CAD build for the part. Positions are in the model's coordinates, mm. A direction names the side the tool comes from. Round coordinates to 2 decimals unless told otherwise and drop trailing zeros. Loops run counter-clockwise (first coordinate to the right, second up) from the corner with the lowest first, then second, coordinate; pieces in that order, holes last.
```python
from build123d import *

# Parameters (mm, degrees)
SKETCH1_W                        = 37
SKETCH1_H                        = 38
BOSS_EXTRUDE1_DEPTH              = 10
SKETCH2_W                        = 34
SKETCH2_H                        = 8
CUT_EXTRUDE1_DEPTH               = 38
CUT_EXTRUDE2_DEPTH               = 3
F_2_05_2_05_DIAMETER_HOLE1_D     = 2.05
F_2_05_2_05_DIAMETER_HOLE1_DEPTH = 10
F_10_0_10_DIAMETER_HOLE1_D       = 10
F_10_0_10_DIAMETER_HOLE1_DEPTH   = 10
F_2_7_2_7_DIAMETER_HOLE1_D       = 2.7
F_2_7_2_7_DIAMETER_HOLE1_DEPTH   = 2
F_2_7_2_7_DIAMETER_HOLE2_D       = 2.7
F_2_7_2_7_DIAMETER_HOLE2_DEPTH   = 2
F_2_7_2_7_DIAMETER_HOLE3_D       = 2.7
F_2_7_2_7_DIAMETER_HOLE3_DEPTH   = 38
CHAMFER1_SIZE                    = 0.15
CHAMFER2_SIZE                    = 0.05
CHAMFER3_SIZE                    = 0.375
FILLET1_R                        = 1.5
FILLET2_R                        = 2


with BuildPart() as part:
    # Sketch1 → Boss-Extrude1 (new body)
    with BuildSketch(Plane(origin=(0, 10, 0), x_dir=(1, 0, 0), z_dir=(0, 1, 0))):
        with Locations((-3.5, 0)):
            Rectangle(SKETCH1_W, SKETCH1_H)
    extrude(amount=-BOSS_EXTRUDE1_DEPTH)

    # Sketch2 → Cut-Extrude1 (cut, through all)
    with BuildSketch(Plane(origin=(15, 0, 0), x_dir=(0, 0, -1), z_dir=(1, 0, 0))):
        with Locations((0, 6)):
            Rectangle(SKETCH2_W, SKETCH2_H)
    extrude(amount=-CUT_EXTRUDE1_DEPTH, mode=Mode.SUBTRACT)

    # Sketch3 → Cut-Extrude2 (cut, through all)
    with BuildSketch(Plane(origin=(0, 2, 0), x_dir=(-1, 0, 0), z_dir=(0, 1, 0))):
        with BuildLine():
            Line((22, -3), (22, 3))
            Line((22, 3), (18, 3))
            ThreePointArc((18, 3), (15, 0), (18, -3))
            Line((18, -3), (22, -3))
        make_face()
    extrude(amount=-CUT_EXTRUDE2_DEPTH, mode=Mode.SUBTRACT)

    # Ø2.05 (2.05) Diameter Hole1
    with Locations(Plane(origin=(0, 0, 0), x_dir=(-1, 0, 0), z_dir=(0, -1, 0))):
        with Locations((-11, 13), (-11, -13), (17, 13), (17, -13), (-11, 4.5), (-4.5, -11), (11, -4.5), (4.5, 11)):
            Hole(F_2_05_2_05_DIAMETER_HOLE1_D / 2, depth=F_2_05_2_05_DIAMETER_HOLE1_DEPTH)

    # Ø10.0 (10) Diameter Hole1
    with Locations(Plane(origin=(0, 0, 0), x_dir=(-1, 0, 0), z_dir=(0, -1, 0))):
        with Locations((0, 0)):
            Hole(F_10_0_10_DIAMETER_HOLE1_D / 2, depth=F_10_0_10_DIAMETER_HOLE1_DEPTH)

    # Ø2.7 (2.7) Diameter Hole1
    with Locations(Plane(origin=(0, 2, 0), x_dir=(1, 0, 0), z_dir=(0, 1, 0))):
        with Locations((11, 0), (7.778174593, 7.778174593), (0, 11), (-7.778174593, 7.778174593), (-11, 0), (-7.778174593, -7.778174593), (0, -11), (7.778174593, -7.778174593), (4.5, 11), (11, -4.5), (-4.5, -11), (-11, 4.5)):
            Hole(F_2_7_2_7_DIAMETER_HOLE1_D / 2, depth=F_2_7_2_7_DIAMETER_HOLE1_DEPTH)

    # Ø2.7 (2.7) Diameter Hole2
    with Locations(Plane.XY.offset(19)):
        with Locations((4, 7.2), (-18, 7.2), (11, 7.2), (-11, 7.2)):
            Hole(F_2_7_2_7_DIAMETER_HOLE2_D / 2, depth=F_2_7_2_7_DIAMETER_HOLE2_DEPTH)

    # Ø2.7 (2.7) Diameter Hole3
    with Locations(Plane(origin=(0, 0, -19), x_dir=(-1, 0, 0), z_dir=(0, 0, -1))):
        with Locations((-4, 7.2), (18, 7.2), (-11, 7.2), (11, 7.2)):
            Hole(F_2_7_2_7_DIAMETER_HOLE3_D / 2, depth=F_2_7_2_7_DIAMETER_HOLE3_DEPTH)

    # Chamfer1
    chamfer1_edges = [part.edges().sort_by_distance(p)[0] for p in [
        (9.128174593, 2, 7.778174593),
        (1.35, 2, 11),
        (-6.428174593, 2, 7.778174593),
        (-9.65, 2, 0),
        (-6.428174593, 2, -7.778174593),
        (1.35, 2, -11),
        (9.128174593, 2, -7.778174593),
        (12.35, 2, 0),
        (-9.65, 7.2, 19),
        (12.35, 7.2, 19),
        (-16.65, 7.2, 19),
        (5.35, 7.2, 19),
        (-12.35, 7.2, -19),
        (9.65, 7.2, -19),
        (-19.35, 7.2, -19),
        (2.65, 7.2, -19),
    ]]
    chamfer(chamfer1_edges, length=CHAMFER1_SIZE)

    # Chamfer2
    chamfer2_edges = [part.edges().sort_by_distance(p)[0] for p in [
        (-9.65, 2, -4.5),
        (-3.15, 2, 11),
        (12.35, 2, 4.5),
        (5.85, 2, -11),
    ]]
    chamfer(chamfer2_edges, length=CHAMFER2_SIZE)

    # Chamfer3
    chamfer3_edges = [part.edges().sort_by_distance(p)[0] for p in [
        (-5.525, 0, -11),
        (-12.025, 0, 4.5),
        (3.475, 0, 11),
        (9.975, 0, -4.5),
        (-18.025, 0, 13),
        (-18.025, 0, -13),
        (9.975, 0, 13),
        (9.975, 0, -13),
    ]]
    chamfer(chamfer3_edges, length=CHAMFER3_SIZE)

    # Fillet1
    fillet1_edges = [part.edges().sort_by_distance(p)[0] for p in [
        (-22, 1, -3),
        (-22, 1, 3),
    ]]
    fillet(fillet1_edges, radius=FILLET1_R)

    # Fillet2
    fillet2_edges = [part.edges().sort_by_distance(p)[0] for p in [
        (-3.5, 0, -19),
        (-22, 10, 18),
        (15, 10, -18),
        (15, 10, 18),
        (-22, 10, -18),
        (-3.5, 0, 19),
    ]]
    fillet(fillet2_edges, radius=FILLET2_R)


solid = part.part
```
Item 1: Two-plate mould, pull along Y, no slides. Class faces 1 (the flat face through (-4, 6, 19)), 2 (the flat face through (-4, 10, -18)), 3 (the cylindrical face through (9.753, 6.683, 17.912)): released by +Y, released by -Y, zero draft, split by the parting line, or undercut.
Answers follow:
face 1: zero draft
face 2: released by +Y
face 3: undercut
Item 2: Cut at C-C, the plane x = 0. Give the cut face in (y, z), plus the area to 3 significant figures.
Answers follow:
outline: (0, -17) arc R2 ccw to (2, -19) - (10, -19) - (10, -17) - (2, -17) - (2, -12.5) - (1.85, -12.35) - (0, -12.35) - close; (0, -9.65) - (1.85, -9.65) - (2, -9.5) - (2, -5) - (0, -5) - close; (0, 5) - (2, 5) - (2, 9.5) - (1.85, 9.65) - (0, 9.65) - close; (0, 12.35) - (1.85, 12.35) - (2, 12.5) - (2, 17) - (10, 17) - (10, 19) - (2, 19) arc R2 ccw to (0, 17) - close
area: 75.4 mm2
Item 3: 3-axis set-ups, long thin cutter, end or side, ignore diameter. For faces 4 (the flat face through (-3, 6, 17)), 5 (the cylindrical face through (-21.57, 0.99, -3.45)), 6 (the cylindrical face through (-5.524, 1.199, -11.045)): which of +Z, -Z, +X, -X, +Y, -Y reach the whole face in a straight line?
Answers follow:
face 4: +X, -X, +Y
face 5: -X, +Y, -Y
face 6: +Y, -Y
Item 4: Cut at D-D, the plane z = 13. Give the cut face in (x, y) (3 decimals), plus the area to 3 significant figures.
Answers follow:
outline: (-22, 0) - (-18.4, 0) - (-18.025, 0.375) - (-18.025, 2) - (-22, 2) - close; (-15.975, 0.375) - (-15.6, 0) - (9.6, 0) - (9.975, 0.375) - (9.975, 2) - (-15.975, 2) - close; (12.025, 0.375) - (12.4, 0) - (15, 0) - (15, 2) - (12.025, 2) - close
area: 65.5 mm2
Item 5: Flat gauge pin, fed straight in: P1, Ø17, axis at x = -11.5, z = 5.5, coming from the +Y side. Where does the tip first touch, or does it go through?
Answers follow:
P1: stops at y = 2
Item 6: Cut at B-B, the plane y = 3.5. Give the cut face in (x, z).
Answers follow:
outline: (-22, -19) - (15, -19) - (15, -17) - (-22, -17) - close; (-22, 17) - (15, 17) - (15, 19) - (-22, 19) - close
Item 7: Probe line 1 (X direction, y = 0.65, z = 11) (3 decimals); line 2 (X direction, y = 1.5, z = -13) (3 decimals); line 3 (Z direction, x = 0, y = 1.2). List the from-to ranges inside material, lowest first.
Answers follow:
line 1: x = -22 to -5.85, -3.15 to -1.35, 1.35 to 3.475, 5.525 to 15
line 2: x = -22 to -18.025, -15.975 to 9.975, 12.025 to 15
line 3: z = -18.83 to -12.35, -9.65 to -5, 5 to 9.65, 12.35 to 18.83
Item 8: Cut at A-A, the plane z = 0. Give the cut face in (x, y).
Answers follow:
outline: (-15, 0) - (-12.35, 0) - (-12.35, 1.85) - (-12.5, 2) - (-15, 2) - close; (-9.65, 0) - (-5, 0) - (-5, 2) - (-9.5, 2) - (-9.65, 1.85) - close; (5, 0) - (9.65, 0) - (9.65, 1.85) - (9.5, 2) - (5, 2) - close; (12.35, 0) - (15, 0) - (15, 2) - (12.5, 2) - (12.35, 1.85) - close
